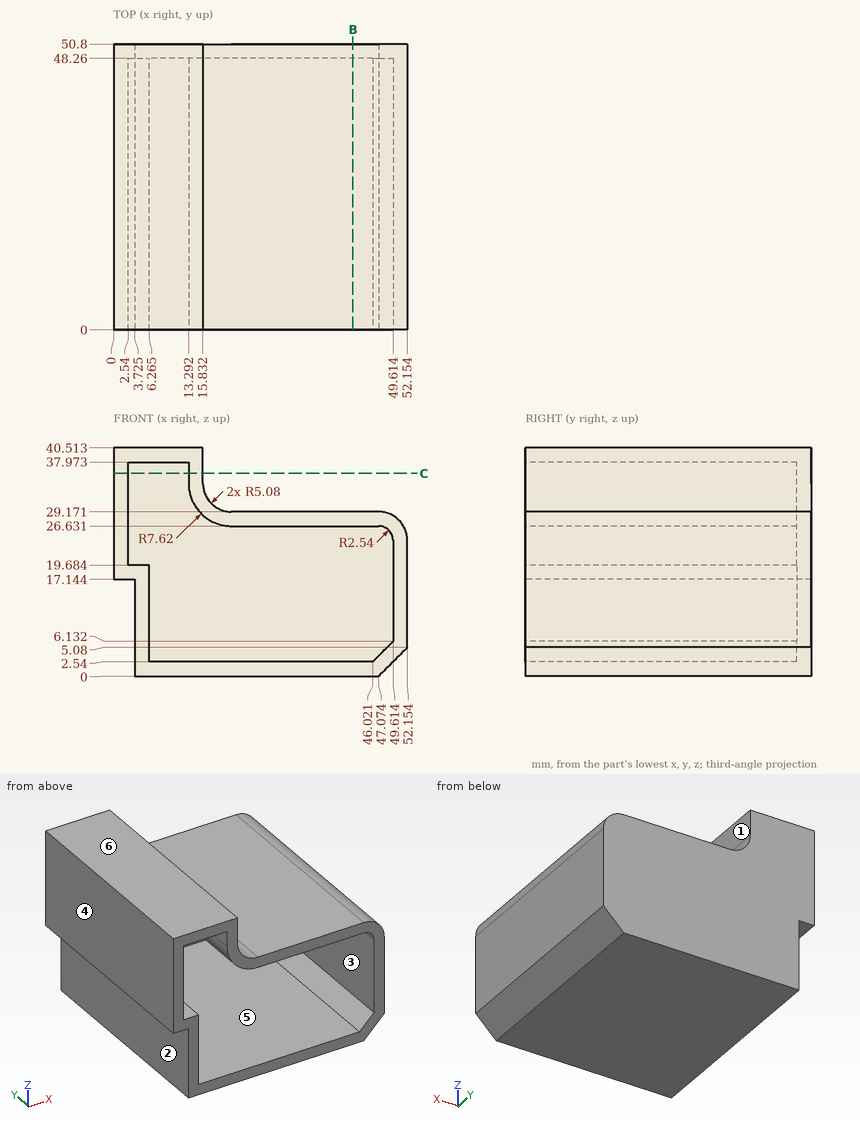
Input: dimensioned drawing with shaded views. Units: mm. Origin: part minimum x, y, z. A direction names the side the tool comes from. Give positions to 0.01 mm unless a question says otherwise; leave off trailing zeros. Order: outer loops, then holes, each group sorted by start corner. A loop starts at its lowest first (then second) coordinate and runs counter-clockwise, first axis right, second up. Notation, with made-up numbers: (-37.5, 16) -> (16.5, 16) arc R22 ccw to (16.5, 53) -> close; hole circle Ø11 at (51, -32). An arc over 180 degrees is marked (long way). Answer as a JSON object with one key per item and string values.
Q1. Access query for the marked faces 1, 2 and 3. Directions: +Z, -Z, +X, -X, +Y, -Y. A direction counts if a zero-diameter tool reaches every point of the face in a straight line with its end or side. Return the directions, or none.
Entries:
{"face 1": "+Z, +X, +Y, -Y", "face 2": "-Z, -X, +Y, -Y", "face 3": "-Y"}
Q2. First-contact query: pin 1 (19 mm diameter, centred on y = 32.5, z = 7.5, fed in from -X) (1 decimal); pin 2 (8 mm diameter, centred on x = 34.5, y = 27.5, fed in from +Z); pin 3 (1.9 mm diameter, centred on x = 1, y = 33.5, fed in from -Z). Flat tips, straight axial feed; report the tip coordinate or a pass-through.
Entries:
{"pin 1": "stops at x = 3.7", "pin 2": "stops at z = 29.17", "pin 3": "stops at z = 17.14"}
Q3. Section B-B (x = 42.5). Output: boundary loops of the cut face in (y, z).
Entries:
{"outline": "(0, 0) -> (50.8, 0) -> (50.8, 29.17) -> (0, 29.17) -> (0, 26.63) -> (48.26, 26.63) -> (48.26, 2.54) -> (0, 2.54) -> close"}
Q4. Material intervals for probe 1 along Z at (x, y) = (20.5, 19.5); probe 2 along X at (y, z) = (44, 23.5); probe 3 along X at (y, z) = (48, 11) (1 decimal), sorted ascending.
Entries:
{"probe 1": "z = 0 to 2.54, 26.64 to 29.19", "probe 2": "x = 0 to 2.54, 49.61 to 52.15", "probe 3": "x = 3.7 to 6.3, 49.6 to 52.2"}
Q5. Section C-C (z = 36). Output: boundary loops of the cut face in (x, y).
Entries:
{"outline": "(0, 0) -> (2.54, 0) -> (2.54, 48.26) -> (13.29, 48.26) -> (13.29, 0) -> (15.83, 0) -> (15.83, 50.8) -> (0, 50.8) -> close"}
Q6. Draft query along X for the marked faces 4, 5 and 6. Return one class per face: released by +X, released by -X, zero draft, split by the parting line, or undercut.
Entries:
{"face 4": "released by -X", "face 5": "undercut", "face 6": "zero draft"}
